from build123d import *

# Parameters (mm, degrees)
SKETCH1_W           = 60
SKETCH1_H           = 30
BOSS_EXTRUDE1_DEPTH = 50
BOSS_EXTRUDE2_DEPTH = 50
SKETCH3_W           = 10
SKETCH3_H           = 30
CUT_EXTRUDE1_DEPTH  = 10
CUT_EXTRUDE2_DEPTH  = 30
CUT_EXTRUDE3_DEPTH  = 10
BOSS_EXTRUDE3_DEPTH = 10


with BuildPart() as part:
    # Sketch1 → Boss-Extrude1 (new body)
    with BuildSketch(Plane.XY):
        with Locations((30, 15)):
            Rectangle(SKETCH1_W, SKETCH1_H)
    extrude(amount=BOSS_EXTRUDE1_DEPTH)

    # Sketch2 → Boss-Extrude2 (add)
    with BuildSketch(Plane.XY.offset(50)):
        Polygon((60, 30), (60, 50), (40, 50), (20, 30), align=None)
    extrude(amount=-BOSS_EXTRUDE2_DEPTH)

    # Sketch3 → Cut-Extrude1 (cut)
    with BuildSketch(Plane.XY.offset(50)):
        with Locations((5, 15)):
            Rectangle(SKETCH3_W, SKETCH3_H)
    extrude(amount=-CUT_EXTRUDE1_DEPTH, mode=Mode.SUBTRACT)

    # Sketch4 → Cut-Extrude2 (cut)
    with BuildSketch(Plane.XY.offset(50)):
        Polygon((40, 50), (20, 30), (40, 30), align=None)
    extrude(amount=-CUT_EXTRUDE2_DEPTH, mode=Mode.SUBTRACT)

    # Sketch5 → Cut-Extrude3 (cut)
    with BuildSketch(Plane(origin=(0, 0, 0), x_dir=(-1, 0, 0), z_dir=(0, 0, -1))):
        Polygon((-20, 30), (-40, 50), (-40, 30), align=None)
    extrude(amount=-CUT_EXTRUDE3_DEPTH, mode=Mode.SUBTRACT)

    # Sketch6 → Boss-Extrude3 (add)
    with BuildSketch(Plane.XY.offset(20)):
        Polygon((20, 30), (40, 30), (40, 50), align=None)
    extrude(amount=BOSS_EXTRUDE3_DEPTH)


solid = part.part
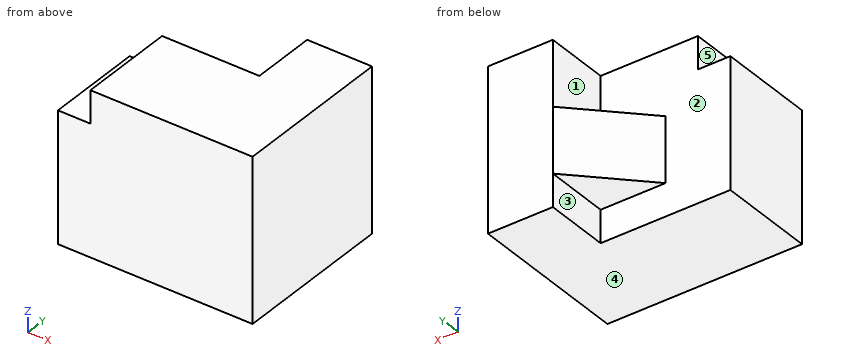
Could you check a few things on this model? Use its own coordinates, in mm. Face numbers are marked on the shaded views. A direction names the side the tool comes from. Round coordinates to 2 decimals unless told otherwise and drop trailing zeros. Order: outer loops, then holes, each group sorted by start corner. A loop starts at its lowest first (then second) coordinate and runs counter-clockwise, first axis right, second up.
(1) I'm going to push flat-ended pins straight in: pin 1 (8 mm diameter, centred on y = 18.5, z = 47, fed in from -X); pin 2 (5 mm diameter, centred on x = 33, z = 28.5, fed in from +Y); pin 3 (8 mm diameter, centred on x = 5.5, y = 19.5, fed in from +Z). Where does each tip first touch, or does it pass through?
Response values:
pin 1: stops at x = 10
pin 2: stops at y = 45.5
pin 3: stops at z = 40
(2) Please list where these lines run through material, in increasing order: line 1 along X through (y, z) = (42.5, 3); line 2 along Y through (x, z) = (18, 36); line 3 along X through (y, z) = (5.5, 44).
Response values:
line 1: x = 40 to 60
line 2: y = 0 to 30
line 3: x = 10 to 60
(3) Imagine slicing it at D-D (z = 44). Write out the boundary of the cut face in (x, y).
Response values:
outline: (10, 0) - (60, 0) - (60, 50) - (40, 50) - (40, 30) - (10, 30) - close
(4) Imagine slicing it at C-C (x = 28.5). Write out the boundary of the cut face in (y, z).
Response values:
outline: (0, 0) - (30, 0) - (30, 10) - (38.5, 10) - (38.5, 30) - (30, 30) - (30, 50) - (0, 50) - close
(5) Which directions (+Z, -Z, +X, -X, +Y, -Y) give clear straight access to the entire face, cutting with the end or side of a thin tool? Please do the marked faces 1, 2, 3, 4 and 5.
Response values:
face 1: +Z, -X, +Y
face 2: -X, +Y
face 3: -Z, -X, +Y
face 4: -Z, +X, -X, +Y, -Y
face 5: +Z, -X, +Y, -Y
(6) Imagine slicing it at A-A (y = 35). Write out the boundary of the cut face in (x, z), plus the area to 3 significant figures.
Response values:
outline: (25, 10) - (40, 10) - (40, 0) - (60, 0) - (60, 50) - (40, 50) - (40, 30) - (25, 30) - close
area: 1,300 mm2
(7) Imagine slicing it at B-B (z = 3). Write out the boundary of the cut face in (x, y).
Response values:
outline: (0, 0) - (60, 0) - (60, 50) - (40, 50) - (40, 30) - (0, 30) - close
